Answer from the drawing. Dimensions are ordinates in mm from the lowest x, y and z of the part. A direction names the side the tool comes from. Round coordinates to 2 decimals unless told otherwise and drop trailing zeros. Write each loop counter-clockwise with the first axis right and the second up, starting at its lowest first coordinate (ties: lowest second). Pieces come first, ordered by that corner, then holes. Notation, with made-up numbers: (2.5, -29.75) - (27.5, -29.75) arc R15 cw to (27.5, -8.75) - close; hole circle Ø4 at (79.25, 11). An arc over 180 degrees is marked (long way). Answer as CSV lines item,"result". Start each with the question number.
1) Find section C-C on z = 26.5. Determine the outline of the cut face in (x, y), then the cut area to 3 significant figures.
2) Find section B-B on y = 36.5. Determine the outline of the cut face in (x, z), then the cut area to 3 significant figures.
3) Find section A-A on x = 33. Determine the outline of the cut face in (y, z), then the cut area to 3 significant figures.
4) Consider line 1 along Y through (x, z) = (34.5, 24); line 2 along Z through (x, y) = (25, 3). Determine where each line is inside the solid, lowest interval first.
5) Find section D-D on x = 53.5. Determine the outline of the cut face in (y, z), then the cut area to 3 significant figures.
6) Which of the six approach directions +Z, -Z, +X, -X, +Y, -Y give full straight-line access (tool end or side, diameter ignored) to the marked faces 1 and 2?
7) For a pull along Y with two mould halves and no side action, classify the marked faces 3, 4 and 5 as +Y half, -Y half, draft (parallel to the pull), parting line (faces both ways), or undercut.
8) Each of these flat-tipped pins is pushed along its axis until it touches: pin 1 (4.5 mm diameter, centred on x = 39.5, y = 4, fed in from +Z); pin 2 (3 mm diameter, centred on y = 38.5, z = 21, fed in from +X). Where does it stop, or does it pass through?
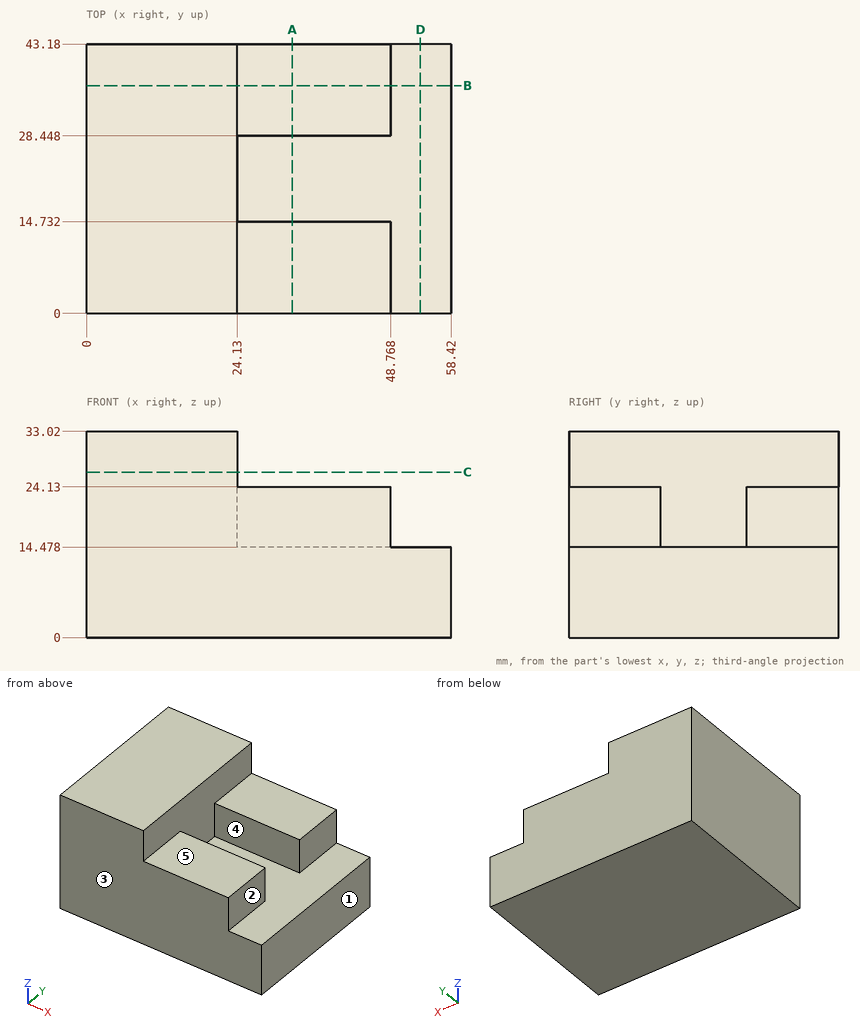
Check values:
1,outline,"(0, 0) - (24.13, 0) - (24.13, 43.18) - (0, 43.18) - close"
1,area,"1,040 mm^2"
2,outline,"(0, 0) - (58.42, 0) - (58.42, 14.48) - (48.77, 14.48) - (48.77, 24.13) - (24.13, 24.13) - (24.13, 33.02) - (0, 33.02) - close"
2,area,"1,530 mm^2"
3,outline,"(0, 0) - (43.18, 0) - (43.18, 24.13) - (28.45, 24.13) - (28.45, 14.48) - (14.73, 14.48) - (14.73, 24.13) - (0, 24.13) - close"
3,area,"910 mm^2"
4,line 1,"y = 0 to 14.73, 28.45 to 43.18"
4,line 2,"z = 0 to 24.13"
5,outline,"(0, 0) - (43.18, 0) - (43.18, 14.48) - (0, 14.48) - close"
5,area,"625 mm^2"
6,face 1,"+Z, -Z, +X, +Y, -Y"
6,face 2,"+Z, +X, +Y, -Y"
7,face 3,"-Y half"
7,face 4,"undercut"
7,face 5,"draft"
8,pin 1,"stops at z = 24.13"
8,pin 2,"stops at x = 48.77"
